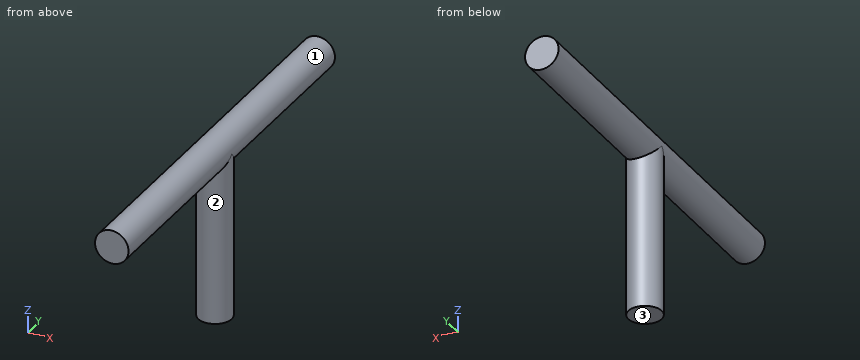
```python
from build123d import *

# Parameters (mm, degrees)
F0_R = 12.7
F6_R = 12.7


with BuildPart() as f4:
    # F4: sweep along a path in F1
    with BuildLine(Plane.YZ) as f4_path:
        Line((0, 0), (0, 127))
    # F0 (on Top) → F4 (sweep)
    with BuildSketch(Plane.XY):
        Circle(F0_R)
    sweep(path=f4_path.line)

    # F7: sweep along a path in F3
    with BuildLine(Plane.XY.offset(127)) as f7_path:
        Line((0, -152.4), (0, 0))
        Line((0, 0), (0, 152.4))
    # F6 (on face) → F7 (sweep)
    with BuildSketch(Plane.XZ.offset(152.4)):
        with Locations((0, 127.014965)):
            Circle(F6_R)
    sweep(path=f7_path.line)


solid = f4.part
```
Source: CAD feature listing. Evaluate the final solid. Frame: model axes, mm. Face numbers are marked on the shaded views. A direction names the side the tool comes from. Round coordinates to 2 decimals unless told otherwise and drop trailing zeros. Order: outer loops, then holes, each group sorted by start corner. A loop starts at its lowest first (then second) coordinate and runs counter-clockwise, first axis right, second up. Notation, with made-up numbers: (-29.5, 41) -> (-25.5, 41) arc R31 ccw to (-25.5, 68) -> close; hole circle Ø2 at (61, 66.25). An arc over 180 degrees is marked (long way). Use CSV: the item, a comma, the result in double quotes.
(1) Ray query, L1, parallel to Z at x = 0.5, y = -30.5; L2, parallel to Z at x = -1, y = -63.5; L3, parallel to Y at x = 0.25, z = 31.5. Return the intervals inside material, ascending.
Report:
L1,"114.32 to 139.71"
L2,"114.35 to 139.68"
L3,"-12.7 to 12.7"
(2) Access query for the marked faces 1, 2 and 3. Directions: +Z, -Z, +X, -X, +Y, -Y. A direction counts if a zero-diameter tool reaches every point of the face in a straight line with its end or side. Return the directions, or none.
Report:
face 1,"none"
face 2,"-Z"
face 3,"-Z, +X, -X, +Y, -Y"
(3) Section C-C on y = -67.5. Return the cut outline in (x, z), and give its area (3 significant figures).
Report:
outline,"circle Ø25.4 at (0, 127.01)"
area,"507 mm^2"
(4) Section B-B on z = 111.5. Return the cut outline in (x, y), and give its area (3 significant figures).
Report:
outline,"circle Ø25.4 at (0, 0)"
area,"507 mm^2"
(5) First-contact query: pin 1 Ø5 at (x, y) = (-9.5, -12) entering from +Z; pin 2 Ø1.5 at (x, y) = (-1.5, -40) entering from -Z; pin 3 Ø1.5 at (x, y) = (-9, -112) entering from +Z. Flat tips, straight axial feed; report the tip coordinate or a pass-through.
Report:
pin 1,"z = 137.61"
pin 2,"z = 114.34"
pin 3,"z = 136.67"
(6) Section A-A on x = 0. Return the cut outline in (y, z), and give its area (3 significant figures).
Report:
outline,"(-152.4, 114.31) -> (-12.7, 114.31) -> (-12.7, 0) -> (12.7, 0) -> (12.7, 114.31) -> (152.4, 114.31) -> (152.4, 139.71) -> (-152.4, 139.71) -> close"
area,"10,600 mm^2"
